Input: part model. Units: mm. Frame: model coordinates. Face numbers are marked on the shaded views. A direction names the side the tool comes from. Coordinates: 2 decimals unless noted, no trailing zeros. Loops run counter-clockwise (first coordinate to the right, second up) from the corner with the lowest first, then second, coordinate; pieces in that order, holes last. Notation, with made-up numbers: (-3.75, 21.5) - (10.25, 21.5) arc R25 ccw to (10.25, 45.5) - close; hole circle Ø5 at (7, 21). An arc over 180 degrees is marked (long way). Use one line per item in the form item = value.
Autodesk Inventor part; units mm, degrees
ref_plane "YZ Plane" through (0, 0, 0) normal (1, 0, 0) x (0, 1, 0)
ref_plane "XZ Plane" through (0, 0, 0) normal (0, 1, 0) x (-1, 0, 0)
ref_plane "XY Plane" through (0, 0, 0) normal (0, 0, 1) x (1, 0, 0)
sketch "Sketch1" plane through (0, 0, 0) normal (0, 1, 0) x (-1, 0, 0)
  circle A0 centre (0, 0) radius 36.83
  dimension "d0" = 73.66
extrude "Extrusion1" add sketch "Sketch1" along normal blind 12.7
fillet "Fillet1" radius 3.175 1 edges at (36.83, 12.7, 0)
sketch "Sketch3" plane through (0, 0, 0) normal (0, -1, 0) x (1, 0, 0)
  circle A0 centre (0, 0) radius 19.05
  dimension "d12" = 38.1
extrude "Extrusion3" cut sketch "Sketch3" against normal blind 6.35
chamfer "Chamfer1" distance 3.175 angle 45 2 edges at (-19.05, 0, 0) (-19.05, 6.35, 0)
sketch "Sketch5" plane through (0, 12.7, 0) normal (0, 1, 0) x (1, 0, 0)
  line L0 (0, 0) -> (0, 27.94)
  point P0 (-26.5725, 8.6339)
  point P1 (-26.5725, 8.6339)
  point P2 (-16.4227, -22.6039)
  point P3 (-16.4227, -22.6039)
  point P4 (16.4227, -22.6039)
  point P5 (16.4227, -22.6039)
  point P6 (26.5725, 8.6339)
  point P7 (26.5725, 8.6339)
  dimension "d18" = 27.94
  dimension "d21" = 360
hole "Hole1" at (0, 12.7, -27.94) at (-26.5725, 12.7, -8.6339) at (-16.4227, 12.7, 22.6039) at (16.4227, 12.7, 22.6039) at (26.5725, 12.7, -8.6339) direction (0, -1, 0) diameter 4 end through all countersink diameter 10 countersink angle 90
properties part number "bearingplate"
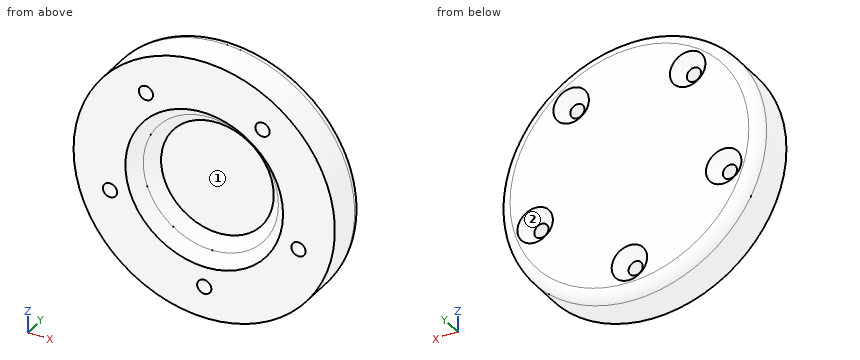
Q1. Set-up query: the marked faces 1 and 2. Return all of +Z, -Z, +X, -X, +Y, -Y with unobstructed straight access to the full face (end or side cutting, diameter ignored); none if empty.
Check values:
face_1 = -Y
face_2 = +Y
Q2. Cut plane D-D, the plane y = 8.25. Return loops of the section in (x, z).
Check values:
outline = circle Ø73.66 at (0, 0); hole circle Ø4 at (-26.57, -8.63); hole circle Ø4 at (-16.42, 22.6); hole circle Ø4 at (0, -27.94); hole circle Ø4 at (16.42, 22.6); hole circle Ø4 at (26.57, -8.63)
Q3. Ray query, line 1 along Z through (x, y) = (0, 3.2); line 2 along Z through (x, y) = (0, 3.75); line 3 along X through (y, z) = (12, 21). Return the intervals inside material, ascending. Write a range as [from, to].
Check values:
line_1 = [-36.83, -29.94], [-25.94, -19.03], [19.03, 36.83]
line_2 = [-36.83, -29.94], [-25.94, -18.48], [18.48, 36.83]
line_3 = [-28.8, -20.41], [-12.43, 12.43], [20.41, 28.8]
Q4. Cut plane C-C, the plane y = 1. Return loops of the section in (x, z), then the cut area to 3 significant figures.
Check values:
outline = circle Ø73.66 at (0, 0); hole circle Ø4 at (-26.57, -8.63); hole circle Ø42.45 at (0, 0); hole circle Ø4 at (-16.42, 22.6); hole circle Ø4 at (0, -27.94); hole circle Ø4 at (16.42, 22.6); hole circle Ø4 at (26.57, -8.63)
area = 2,780 mm²
Q5. First-contact query: P1, Ø6, axis at x = 3.5, y = 8.5, coming from the +Z side; P2, Ø23, axis at x = 0, z = 0, coming from the -Y side; P3, Ø2, axis at y = 7, z = 7.5, coming from the -X side. Flat tips, straight axial feed; report the tip coordinate or a pass-through.
Check values:
P1 = 36.83
P2 = 6.35
P3 = -36.25
